Check sheet for the modelled part. Datum: model origin and axes. Units: mm. A direction names the side the tool comes from. Coordinates: 2 decimals unless noted, no trailing zeros. Loops run counter-clockwise (first coordinate to the right, second up) from the corner with the lowest first, then second, coordinate; pieces in that order, holes last.
Autodesk Inventor part; units mm, degrees
ref_plane "YZ Plane" through (0, 0, 0) normal (1, 0, 0) x (0, 1, 0)
ref_plane "XZ Plane" through (0, 0, 0) normal (0, 1, 0) x (-1, 0, 0)
ref_plane "XY Plane" through (0, 0, 0) normal (0, 0, 1) x (1, 0, 0)
sketch "Sketch1" plane through (0, 0, 0) normal (0, 1, 0) x (-1, 0, 0)
  line L0 (-15.1925, 10.3416) -> (7.8075, 10.3416)
  line L1 (7.8075, 10.3416) -> (7.8075, -34.6584)
  line L2 (7.8075, -34.6584) -> (-15.1925, -34.6584)
  line L3 (-15.1925, -34.6584) -> (-15.1925, -19.6584)
  line L4 (-15.1925, 10.3416) -> (-15.1925, -4.6584)
  line L5 (-15.1925, -4.6584) -> (-5.1925, -4.6584)
  line L6 (-5.1925, -4.6584) -> (-5.1925, -19.6584)
  line L7 (-5.1925, -19.6584) -> (-15.1925, -19.6584)
  circle A0 centre (-12.1925, -31.6584) radius 1.5
  circle A1 centre (3.8075, 7.3416) radius 1.5
  point P0 (0, 0)
  dimension "d0" = 23
  dimension "d1" = 45
  dimension "d2" = 15
  dimension "d3" = 15
  dimension "d4" = 10
  dimension "d5" = 3
  dimension "d6" = 3
  dimension "d7" = 3
  dimension "d8" = 3
  dimension "d10" = 3
  dimension "d23" = 23
  dimension "d24" = 19
extrude "Extrusion1" add sketch "Sketch1" along normal blind 3
sketch "Sketch2" plane through (0, 3, 0) normal (0, 1, 0) x (1, 0, 0)
  line L0 (-7.8075, 34.6584) -> (-7.8075, -10.3416)
  line L1 (-7.8075, -0.3416) -> (-4.8075, -0.3416)
  line L2 (-4.8075, -0.3416) -> (-4.8075, 24.6584)
  line L3 (-4.8075, 24.6584) -> (-7.8075, 24.6584)
  line L4 (-7.8075, 24.6584) -> (-7.8075, -0.3416)
  line L5 (15.1925, 34.6584) -> (-7.8075, 34.6584)
  line L6 (-7.8075, -10.3416) -> (15.1925, -10.3416)
  point P0 (0, 0)
  dimension "d13" = 10
  dimension "d14" = 10
  dimension "d15" = 3
extrude "Extrusion2" add sketch "Sketch2" along normal blind 20
sketch "Sketch3" plane through (-7.8075, 0, -34.6584) normal (-1, 0, 0) x (0, 0, 1)
  circle A0 centre (22.5, 13) radius 1.5
  line L0 (10, 23) -> (35, 23)
  line L1 (10, 3) -> (10, 23)
  point P0 (34.6584, 0)
  dimension "d18" = 10
  dimension "d19" = 12.5
  dimension "d20" = 3
extrude "Extrusion3" cut sketch "Sketch3" against normal up to surface (3 mm away)
properties part number "support-srf04"
(1) Gauge pin test, flat ends, axial feed: P1, Ø1.5, axis at y = 13.5, z = -9, coming from the +X side; P2, Ø0.9, axis at x = -7, y = 15, coming from the -Z side; P3, Ø4, axis at x = 10, z = 1.5, coming from the +Y side; P4, Ø2, axis at y = 12.5, z = -25.5, coming from the -X side. Record the tip position at first contact, or that the pin passes through.
(2) Section check A-A, the plane y = 13. Enter the section's corners in (x, z).
(3) Section check D-D, the plane x = -6. Enter the section's corners in (y, z), plus the area to 3 significant figures.
(4) Section check C-C, the plane z = -18. Enter the section's corners in (x, y).
(5) Section check B-B, the plane x = -3.5. Enter the section's corners in (y, z), plus the area to 3 significant figures.
(6) Set-up check for faces 1 (the face through (10, 1, -4.658)), 2 (the face through (-6, 13, -24.658)), 3 (the face through (-4.808, 11, -12)), 4 (the face through (-6, 13, 0.342)): record each of +Z, -Z, +X, -X, +Y, -Y from which the full face is reachable in a straight line by a thin tool's end or side.
(7) Scan lines: line 1 along X through (y, z) = (9.5, -18); line 2 along Y through (x, z) = (11.5, -20.5). Record each from-to range of solid material in increasing order.
(8) Draft check along X on faces 5 (the face through (-3.612, 1.479, 5.854)), 6 (the face through (4, 1, -34.658)), 7 (the face through (5.192, 1, -12)). Enter one of: pulls with the +X half, pulls with the -X half, needs draft (parallel to the pull), parting line crosses it, or undercut.
Determined:
1. P1: stops at x = -4.81
1. P2: stops at z = -24.66
1. P3: stops at y = 3
1. P4: stops at x = -7.81
2. outline: (-7.81, -24.66) - (-4.81, -24.66) - (-4.81, -13.66) - (-7.81, -13.66) - close; (-7.81, -10.66) - (-4.81, -10.66) - (-4.81, 0.34) - (-7.81, 0.34) - close
3. outline: (0, -34.66) - (3, -34.66) - (3, -24.66) - (23, -24.66) - (23, 0.34) - (3, 0.34) - (3, 10.34) - (0, 10.34) - close; hole circle Ø3 at (13, -12.16)
3. area: 628 mm2
4. outline: (-7.81, 0) - (5.19, 0) - (5.19, 3) - (-4.81, 3) - (-4.81, 23) - (-7.81, 23) - close
5. outline: (0, -34.66) - (3, -34.66) - (3, 5.87) - (0, 5.87) - close; (0, 8.81) - (3, 8.81) - (3, 10.34) - (0, 10.34) - close
5. area: 126 mm2
6. face 1: +X, +Y, -Y
6. face 2: -Z, +X, -X, +Y
6. face 3: +Z, -Z, +X, +Y
6. face 4: +Z, +X, -X, +Y
7. line 1: x = -7.81 to -4.81
7. line 2: y = 0 to 3
8. face 5: undercut
8. face 6: needs draft
8. face 7: pulls with the +X half
